Geometry check sheet. Reference: the model listing, model coordinates, mm. Give positions to 0.01 mm unless a question says otherwise; leave off trailing zeros. Loops run counter-clockwise (first coordinate to the right, second up) from the corner with the lowest first, then second, coordinate; pieces in that order, holes last. Notation, with made-up numbers: (84, 58) -> (93, 58) arc R13 ccw to (93, 68) -> close; hole circle Ø4 at (-9.75, 9). An arc over 180 degrees is marked (long way). Write item = value, one per line.
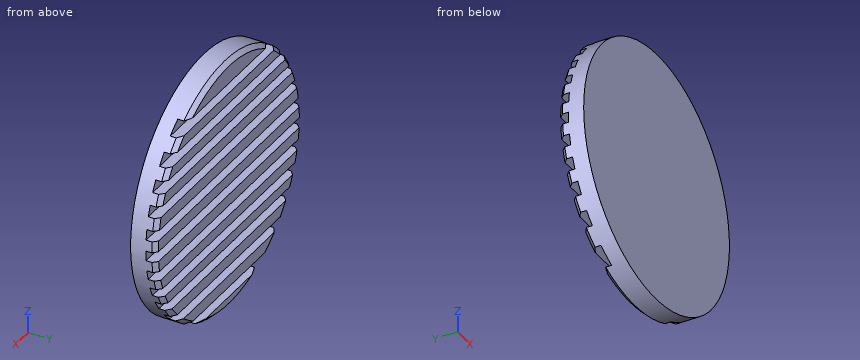
Autodesk Inventor part; units mm, degrees
ref_plane "YZ Plane" through (0, 0, 0) normal (1, 0, 0) x (0, 1, 0)
ref_plane "XZ Plane" through (0, 0, 0) normal (0, 1, 0) x (-1, 0, 0)
ref_plane "XY Plane" through (0, 0, 0) normal (0, 0, 1) x (1, 0, 0)
sketch "Sketch1" plane through (0, 0, 0) normal (0, 1, 0) x (-1, 0, 0)
  circle A0 centre (0, 0) radius 250
  dimension "d0" = 500
extrude "Extrusion1" add sketch "Sketch1" along normal blind 50
chamfer "Chamfer1" distance 8.35 angle 45 1 edges at (250, 50, 0)
sketch "Sketch2" plane through (0, 50, 0) normal (0, 1, 0) x (1, 0, 0)
  circle A0 centre (0, 0) radius 250
  line L0 (-269.1595, 0) -> (277.2847, 0)
  line L1 (277.2847, 0) -> (277.2847, 20)
  line L2 (277.2847, 20) -> (-269.1595, 20)
  line L3 (-269.1595, 20) -> (-269.1595, 0)
  line L4 (-257.5823, 42.3509) -> (264.9356, 42.3509)
  line L5 (264.9356, 42.3509) -> (264.9356, 62.3509)
  line L6 (264.9356, 62.3509) -> (-257.5823, 62.3509)
  line L7 (-257.5823, 62.3509) -> (-257.5823, 42.3509)
  line L8 (-250, 83.257) -> (254.1302, 83.257)
  line L9 (254.1302, 83.257) -> (254.1302, 103.257)
  line L10 (254.1302, 103.257) -> (-250, 103.257)
  line L11 (-250, 103.257) -> (-250, 83.257)
  line L12 (-232.1124, 122.6195) -> (241.7812, 122.6195)
  line L13 (241.7812, 122.6195) -> (241.7812, 142.6195)
  line L14 (241.7812, 142.6195) -> (-232.1124, 142.6195)
  line L15 (-232.1124, 142.6195) -> (-232.1124, 122.6195)
  line L16 (-202.0117, 165.0693) -> (241.7812, 165.0693)
  line L17 (241.7812, 165.0693) -> (241.7812, 185.0693)
  line L18 (241.7812, 185.0693) -> (-202.0117, 185.0693)
  line L19 (-202.0117, 185.0693) -> (-202.0117, 165.0693)
  line L20 (-151.8438, 208.2908) -> (197.016, 208.2908)
  line L21 (197.016, 208.2908) -> (197.016, 228.2908)
  line L22 (197.016, 228.2908) -> (-151.8438, 228.2908)
  line L23 (-151.8438, 228.2908) -> (-151.8438, 208.2908)
  line L24 (-257.5823, -21.7096) -> (271.882, -21.7096)
  line L25 (271.882, -21.7096) -> (271.882, -41.7096)
  line L26 (271.882, -41.7096) -> (-257.5823, -41.7096)
  line L27 (-257.5823, -41.7096) -> (-257.5823, -21.7096)
  line L28 (-250, -64.9312) -> (264.9356, -64.9312)
  line L29 (264.9356, -64.9312) -> (264.9356, -84.9312)
  line L30 (264.9356, -84.9312) -> (-250, -84.9312)
  line L31 (-250, -84.9312) -> (-250, -64.9312)
  line L32 (-236.7433, -105.8373) -> (254.1302, -105.8373)
  line L33 (254.1302, -105.8373) -> (254.1302, -125.8373)
  line L34 (254.1302, -125.8373) -> (-236.7433, -125.8373)
  line L35 (-236.7433, -125.8373) -> (-236.7433, -105.8373)
  line L36 (-215.9043, -145.9716) -> (224.8013, -145.9716)
  line L37 (224.8013, -145.9716) -> (224.8013, -165.9716)
  line L38 (224.8013, -165.9716) -> (-215.9043, -165.9716)
  line L39 (-215.9043, -165.9716) -> (-215.9043, -145.9716)
  line L40 (-185.0318, -186.8778) -> (209.3651, -186.8778)
  line L41 (209.3651, -186.8778) -> (209.3651, -206.8778)
  line L42 (209.3651, -206.8778) -> (-185.0318, -206.8778)
  line L43 (-185.0318, -206.8778) -> (-185.0318, -186.8778)
  dimension "d6" = 20
  dimension "d7" = 20
  dimension "d8" = 20
  dimension "d9" = 20
  dimension "d10" = 20
  dimension "d11" = 20
  dimension "d12" = 20
  dimension "d13" = 20
  dimension "d14" = 20
  dimension "d15" = 20
  dimension "d16" = 20
extrude "Extrusion2" cut sketch "Sketch2" against normal blind 20 contours L0 A0 L2 | A0 L2 L1 L0 | L24 L25 L26 A0 | A0 L26 L24 | L0 L3 L2 A0 | L4 A0 L6 | A0 L6 L5 L4 | A0 L26 L27 L24 | L4 L7 L6 A0 | L28 L29 L30 A0 | A0 L30 L28 | L8 A0 L10 | A0 L10 L9 L8 | A0 L30 L31 L28 | L8 L11 L10 A0 | L32 L33 L34 A0 | A0 L34 L32 | L12 A0 L14 | A0 L14 L13 L12 | A0 L34 L35 L32 | L12 L15 L14 A0 | L36 L37 L38 A0 | A0 L38 L36 | L16 A0 L18 | A0 L18 L17 L16 | A0 L38 L39 L36 | L16 L19 L18 A0 | L40 L41 L42 A0 | A0 L42 L40 | L20 A0 L22 | A0 L22 L21 L20 | A0 L42 L43 L40 | L20 L23 L22 A0
properties part number "MachiningBase"
Item 1: Section check B-B, the plane z = -215. Record the cut outline in (x, y).
Answer:
outline = (-127.57, 0) -> (127.57, 0) -> (127.57, 30) -> (-127.57, 30) -> close
Item 2: Thickness scan on L1, parallel to Z at x = -221.5, y = 32; L2, parallel to Y at x = -98.5, z = -47.5; L3, parallel to X at y = 28.5, z = -8. Record the ranges inside material, lowest first. Write a range as [from, to].
Answer:
L1 = [-115.92, -103.26], [-83.26, -62.35], [-42.35, -20], [0, 21.71], [41.71, 64.93], [84.93, 105.84]
L2 = [0, 30]
L3 = [-249.87, 249.87]
Item 3: Gauge pin test, flat ends, axial feed: pin 1 (1 mm diameter, centred on x = -129.5, y = 26, fed in from -Z); pin 2 (16 mm diameter, centred on x = -4.5, z = 201, fed in from +Y); pin 3 (10 mm diameter, centred on x = 19, y = 35.5, fed in from +Z); pin 4 (10 mm diameter, centred on x = 51.5, z = 112, fed in from +Y). Record the tip position at first contact, or that the pin passes through.
Answer:
pin_1 = -214.15
pin_2 = 50
pin_3 = 249.61
pin_4 = 30
Item 4: Section check A-A, the plane y = 10.5. Record the cut outline in (x, z).
Answer:
outline = circle Ø500 at (0, 0)
